Design review of the part shown in the three views and the two pictorial views. Dimensions are in mm from the part's minimum x, y and z. Round coordinates to 2 decimals unless told otherwise and drop trailing zeros. Write each loop counter-clockwise with the first axis right and the second up, starting at its lowest first coordinate (ties: lowest second). Pieces come first, ordered by that corner, then holes. Notation, with made-up numbers: (17.25, 58.5) - (52.25, 58.5) arc R15 cw to (52.25, 85.5) - close; hole circle Ø11 at (42, 88). An arc over 180 degrees is marked (long way). One line per item, written item: value. Start each with the question number.
Q1. Add section B-B on z = 77. Write out the cut boundary in (x, y).
Q2. Add section A-A on y = 10. Write out the cut boundary in (x, z).
Q3. Add section C-C on y = 34.5. Write out the cut boundary in (x, z), and give its area (3 significant figures).
Q4. Mouldability with a two-part tool opening along Y and no side actions: class the marked faces 1 and 2 as +Y half, -Y half, draft (parallel to the pull), parting line (faces both ways), or undercut.
Q5. For probe 1 along Y at (x, z) = (7, 103) (1 decimal); probe 2 along Y at (x, z) = (8.25, 18.5); probe 3 along Y at (x, z) = (3.75, 41.5) (1 decimal), list the stretches that pass through material, from the lowest coordinate up.
Q6. Clearance check with flat-ended pins moving along their axes: pin 1 Ø2.5 at (y, z) = (2, 43.5) entering from +X; pin 2 Ø1.5 at (x, z) = (8.5, 33.5) entering from -Y (1 decimal); pin 3 Ø5 at (x, z) = (8.5, 47) entering from -Y. State where each tip first meets the part, or that it passes through.
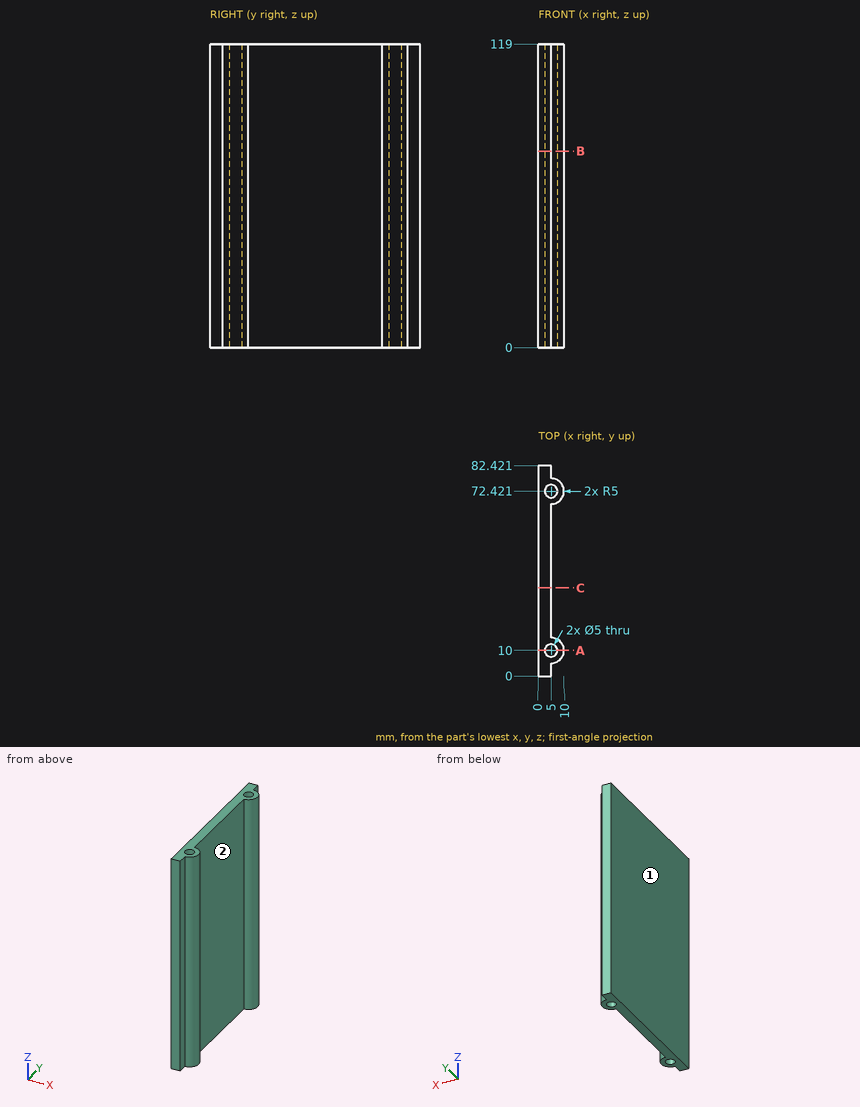
Result set:
1. outline: (0, 0) - (5, 0) - (5, 5) arc R5 ccw to (5, 15) - (5, 67.42) arc R5 ccw to (5, 77.42) - (5, 82.42) - (0, 82.42) - close; hole circle Ø5 at (5, 10); hole circle Ø5 at (5, 72.42)
2. outline: (0, 0) - (2.5, 0) - (2.5, 119) - (0, 119) - close; (7.5, 0) - (10, 0) - (10, 119) - (7.5, 119) - close
3. outline: (0, 0) - (5, 0) - (5, 119) - (0, 119) - close
3. area: 595 mm^2
4. face 1: draft
4. face 2: undercut
5. probe 1: y = 5.4 to 8.5, 11.5 to 14.6, 67.8 to 70.9, 73.9 to 77
5. probe 2: y = 6.2 to 13.8, 68.62 to 76.22
5. probe 3: y = 0 to 7.8, 12.2 to 70.3, 74.6 to 82.4
6. pin 1: stops at x = 5
6. pin 2: stops at y = 5.8
6. pin 3: stops at y = 5.1
